The model under review builds one solid part; all positions refer to its coordinate system, in mm. Coordinates: 2 decimals unless noted, no trailing zeros. Write each loop counter-clockwise with the first axis right and the second up, starting at its lowest first coordinate (ties: lowest second). Pieces come first, ordered by that corner, then holes. Notation, with made-up numbers: (82.5, -30.5) - (98.5, -30.5) arc R34 ccw to (98.5, 4.5) - close; hole circle Ø11 at (10, 48). An arc over 180 degrees is marked (long way). Return JSON: item names as keys, results as strings. Group by question number.
(1) We need section A-A on x = 0. State the section outline as (y, z) points.
(2) We need section D-D on x = 15.5. State the section outline as (y, z) points.
(3) Draft analysis for pull direction X (two halves, no side actions). For faces 1 (the face through (9, 0, -9)), 2 (the face through (17.5, 0.2, -17.5)), 3 (the face through (13.926, 0.197, -15.004)), state which applies: released by +X, released by -X, zero draft, split by the parting line, or undercut.
(4) We need section B-B on y = 0.2. State the section outline as (x, z) points.
(5) We need section C-C on z = 0. State the section outline as (x, y) points, then the cut area to 3 significant figures.
(6) To check wall thickness, follow L1, parallel to Z at x = 15.5, y = 0.15; L2, parallel to X at y = 0.1, z = -16; L3, parallel to Z at x = 15, y = 0.1. State the ranges of each line that lie inside material, in increasing order. Write a range as from..to.
```python
from build123d import *

# Parameters (mm, degrees)
SKETCH1_W           = 41
SKETCH1_H           = 41
SKETCH1_R           = 11.25
SKETCH1_R_2         = 1.65
BOSS_EXTRUDE1_DEPTH = 0.4
CHAMFER1_SIZE       = 6


with BuildPart() as part:
    # Sketch1 → Boss-Extrude1 (new body)
    with BuildSketch(Plane(origin=(0, 0, 0), x_dir=(-1, 0, 0), z_dir=(0, 1, 0))):
        Rectangle(SKETCH1_W, SKETCH1_H)
        Circle(SKETCH1_R, mode=Mode.SUBTRACT)
        with Locations((15.5, 15.5)):
            Circle(SKETCH1_R_2, mode=Mode.SUBTRACT)
        with Locations((-15.5, 15.5)):
            Circle(SKETCH1_R_2, mode=Mode.SUBTRACT)
        with Locations((-15.5, -15.5)):
            Circle(SKETCH1_R_2, mode=Mode.SUBTRACT)
        with Locations((15.5, -15.5)):
            Circle(SKETCH1_R_2, mode=Mode.SUBTRACT)
    extrude(amount=BOSS_EXTRUDE1_DEPTH)

    # Chamfer1
    chamfer1_edges = [part.edges().sort_by_distance(p)[0] for p in [
        (-20.5, 0.2, -20.5),
        (20.5, 0.2, -20.5),
        (20.5, 0.2, 20.5),
        (-20.5, 0.2, 20.5),
    ]]
    chamfer(chamfer1_edges, length=CHAMFER1_SIZE)


solid = part.part
```
Ans:
{
 "1": {"outline": "(0, -20.5) - (0.4, -20.5) - (0.4, -11.25) - (0, -11.25) - close; (0, 11.25) - (0.4, 11.25) - (0.4, 20.5) - (0, 20.5) - close"},
 "2": {"outline": "(0, -19.5) - (0.4, -19.5) - (0.4, -17.15) - (0, -17.15) - close; (0, -13.85) - (0.4, -13.85) - (0.4, 13.85) - (0, 13.85) - close; (0, 17.15) - (0.4, 17.15) - (0.4, 19.5) - (0, 19.5) - close"},
 "3": {"face 1": "zero draft", "face 2": "released by +X", "face 3": "undercut"},
 "4": {"outline": "(-20.5, -14.5) - (-14.5, -20.5) - (14.5, -20.5) - (20.5, -14.5) - (20.5, 14.5) - (14.5, 20.5) - (-14.5, 20.5) - (-20.5, 14.5) - close; hole circle Ø3.3 at (-15.5, -15.5); hole circle Ø3.3 at (-15.5, 15.5); hole circle Ø22.5 at (0, 0); hole circle Ø3.3 at (15.5, -15.5); hole circle Ø3.3 at (15.5, 15.5)"},
 "5": {"outline": "(-20.5, 0) - (-11.25, 0) - (-11.25, 0.4) - (-20.5, 0.4) - close; (11.25, 0) - (20.5, 0) - (20.5, 0.4) - (11.25, 0.4) - close", "area": "7.40 mm²"},
 "6": {"L1": "-19.5..-17.15, -13.85..13.85, 17.15..19.5", "L2": "-19..-17.07, -13.93..13.93, 17.07..19", "L3": "-20..-17.07, -13.93..13.93, 17.07..20"}
}
